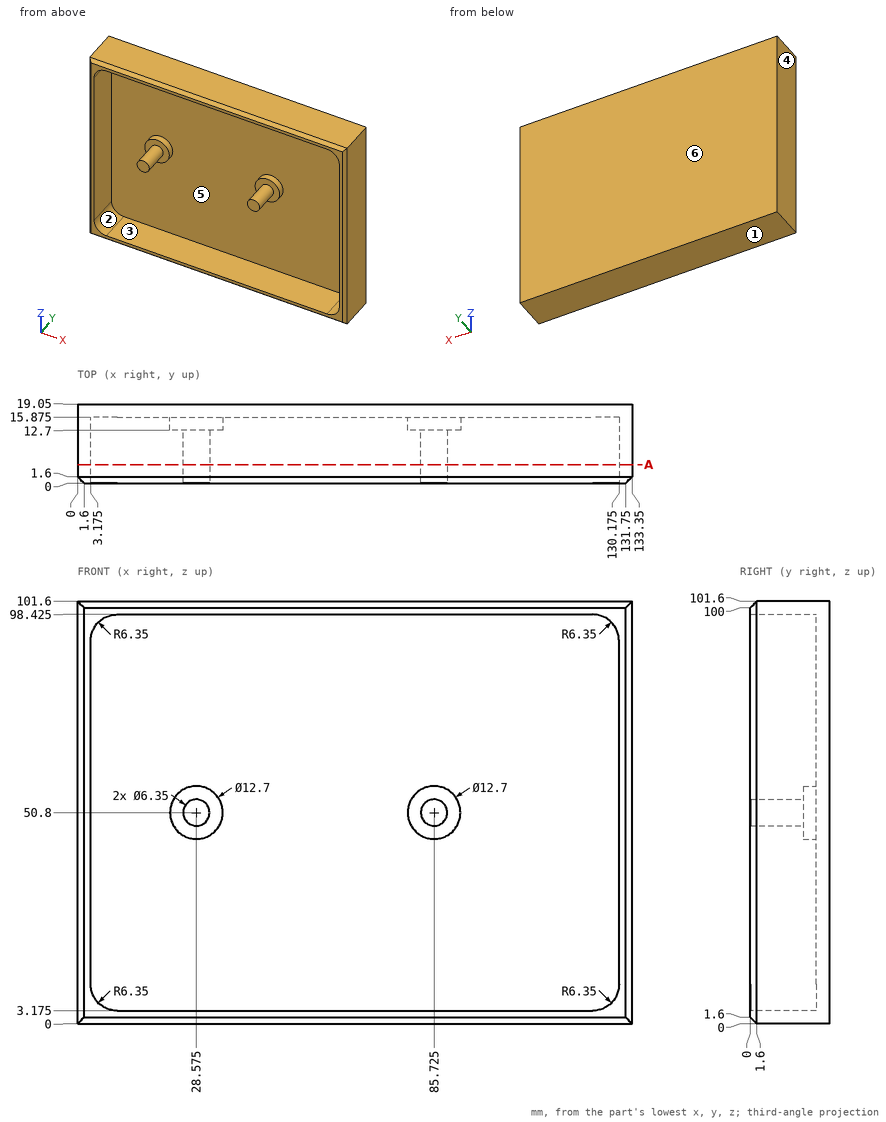
The drawing under review shows one solid part. Ordinate dimensions are in mm from its lowest x, y, z. A direction names the side the tool comes from. Coordinates: 2 decimals unless noted, no trailing zeros. Write each loop counter-clockwise with the first axis right and the second up, starting at its lowest first coordinate (ties: lowest second). Pieces come first, ordered by that corner, then holes. Notation, with made-up numbers: (-37.75, 36.5) - (8.25, 36.5) arc R15 ccw to (8.25, 44.5) - close; hole circle Ø8 at (77, 54). An arc over 180 degrees is marked (long way). Use one line per item in the form item = value.
Q1. For probe 1 along X at (y, z) = (15.75, 88) (3 decimals); probe 2 along Z at (x, y) = (17, 4.25) (3 decimals); probe 3 along Y at (x, z) = (57, 95.5) (3 decimals), list the stretches that pass through material, from the lowest coordinate up.
Taken from the geometry:
probe_1 = 0 to 3.175, 130.175 to 133.35
probe_2 = 0 to 3.175, 98.425 to 101.6
probe_3 = 15.875 to 19.05
Q2. Consider section A-A (y = 4.5). Write out the cut boundary in (x, z) (3 decimals), plus the area to 3 significant figures.
Taken from the geometry:
outline = (0, 0) - (133.35, 0) - (133.35, 101.6) - (0, 101.6) - close; circle Ø6.35 at (28.575, 50.8); circle Ø6.35 at (85.725, 50.8); hole (3.175, 9.525) arc R6.35 ccw to (9.525, 3.175) - (123.825, 3.175) arc R6.35 ccw to (130.175, 9.525) - (130.175, 92.075) arc R6.35 ccw to (123.825, 98.425) - (9.525, 98.425) arc R6.35 ccw to (3.175, 92.075) - close
area = 1,550 mm^2
Q3. Insertion check: pin 1 Ø5 at (x, z) = (106.5, 90) entering from -Y (3 decimals); pin 2 Ø4 at (x, z) = (93, 48) entering from -Y. Each pin has a flat end and moves straight along its axis. Give the tip position at first contact, or say it passes through.
Taken from the geometry:
pin_1 = 15.875
pin_2 = 12.7
Q4. The part is to be moulded in two halves that separate along X. For the marked faces 1, 2, 3 and 4, say which applies: +X half, -X half, draft (parallel to the pull), parting line (faces both ways), or undercut.
Taken from the geometry:
face_1 = draft
face_2 = undercut
face_3 = undercut
face_4 = -X half
Q5. Machinability: for the marked faces 5 and 6, which of the approach directions +Z, -Z, +X, -X, +Y, -Y give a long, thin tool a straight path to every point of the face, cutting with its end or side? Answer none if there is none.
Taken from the geometry:
face_5 = -Y
face_6 = +Z, -Z, +X, -X, +Y
